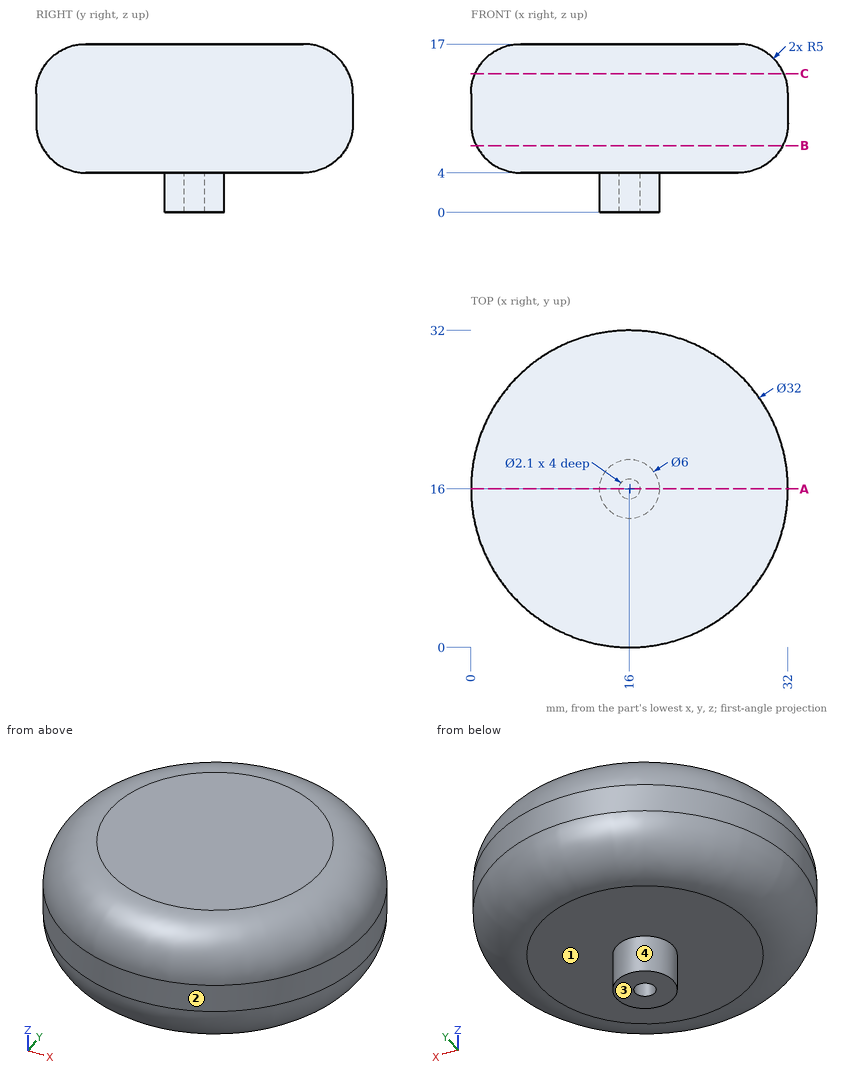
Answer from the drawing. Dimensions are ordinates in mm from the lowest x, y and z of the part. A direction names the side the tool comes from. Give positions to 0.01 mm unless a question says otherwise; leave off trailing zeros. Loops run counter-clockwise (first coordinate to the right, second up) from the corner with the lowest first, then second, coordinate; pieces in that order, holes last. Notation, with made-up numbers: (47.5, 32) -> (73.5, 32) arc R24 cw to (73.5, 45) -> close; hole circle Ø3 at (3.25, 29). An arc over 180 degrees is marked (long way). Answer as CSV lines item,"result".
Item 1: Each of these flat-tipped pins is pushed along its axis until it touches: pin 1 (10 mm diameter, centred on x = 6, z = 10, fed in from +Y); pin 2 (3 mm diameter, centred on y = 22.5, z = 14, fed in from +X); pin 3 (1.5 mm diameter, centred on x = 14.5, z = 12.5, fed in from +Y). Where does it stop, or does it pass through?
Returned:
pin 1,"stops at y = 31.2"
pin 2,"stops at x = 30.97"
pin 3,"stops at y = 31.98"
Item 2: Find section B-B on z = 6.75. Give the vertices of the cut face in (x, y), plus the area to 3 significant figures.
Returned:
outline,"circle Ø30.93 at (16, 16)"
area,"751 mm²"
Item 3: Consider line 1 (X direction, y = 16, z = 1.4); line 2 (Z direction, x = 10, y = 13). Determine where each line is inside the solid, lowest interval first. Write a range as [from, to].
Returned:
line 1,"x = [13, 14.95], [17.05, 19]"
line 2,"z = [4, 17]"
Item 4: Determine the mould class of the marked faces 1 and 2 for opening direction Y: +Y half, -Y half, draft (parallel to the pull), parting line (faces both ways), or undercut.
Returned:
face 1,"draft"
face 2,"parting line"
Item 5: Find section C-C on z = 14. Give the vertices of the cut face in (x, y).
Returned:
outline,"circle Ø31.17 at (16, 16)"
Item 6: For the marked faces 3 and 4, determine the directions among +Z, -Z, +X, -X, +Y, -Y from which every point of the face is accessible in a straight line to the end or side of a thin tool.
Returned:
face 3,"-Z, +X, -X, +Y, -Y"
face 4,"-Z"
Item 7: Find section A-A on y = 16. Give the vertices of the cut face in (x, z), plus the area to 3 significant figures.
Returned:
outline,"(0, 9) arc R5 ccw to (5, 4) -> (13, 4) -> (13, 0) -> (14.95, 0) -> (14.95, 4) -> (17.05, 4) -> (17.05, 0) -> (19, 0) -> (19, 4) -> (27, 4) arc R5 ccw to (32, 9) -> (32, 12) arc R5 ccw to (27, 17) -> (5, 17) arc R5 ccw to (0, 12) -> close"
area,"410 mm²"
